```python
from build123d import *

# Parameters (mm, degrees)
BOSS_EXTRUDE1_DEPTH  = 1.5875
M8_CLEARANCE_HOLE1_D = 8.4


with BuildPart() as part:
    # Sketch1 → Boss-Extrude1 (new body)
    with BuildSketch(Plane(origin=(0, 0, 0), x_dir=(0, 0, -1), z_dir=(1, 0, 0))):
        with BuildLine():
            Line((-9.466844547, 1.05094211), (-8.132830894, 13.067683806))
            Line((-8.132830894, 13.067683806), (-6.55502347, 12.892526787))
            Line((-6.55502347, 12.892526787), (-4.453139249, 31.826215882))
            Line((-4.453139249, 31.826215882), (-6.030946674, 32.0013729))
            Line((-6.030946674, 32.0013729), (-4.696933021, 44.018114595))
            Line((-4.696933021, 44.018114595), (30.078862848, 47.728850174))
            ThreePointArc((30.078862848, 47.728850174), (38.60002065, 37.058807525), (51.869269545, 40.281690423))
            Line((51.869269545, 40.281690423), (35.966414021, 23.714419941))
            Line((35.966414021, 23.714419941), (34.821152107, 24.813752193))
            Line((34.821152107, 24.813752193), (21.629165093, 11.070609225))
            Line((21.629165093, 11.070609225), (22.774427007, 9.971276974))
            Line((22.774427007, 9.971276974), (6.871571484, -6.595993507))
            ThreePointArc((6.871571484, -6.595993507), (-4.037668467, -8.626868397), (-9.466844547, 1.05094211))
        make_face()
    extrude(amount=BOSS_EXTRUDE1_DEPTH)

    # M8 Clearance Hole1 (through all)
    with Locations(Plane(origin=(1.5875, 0, 0), x_dir=(0, 0, -1), z_dir=(1, 0, 0))):
        with Locations((0, 0)):
            Hole(M8_CLEARANCE_HOLE1_D / 2)


solid = part.part
```
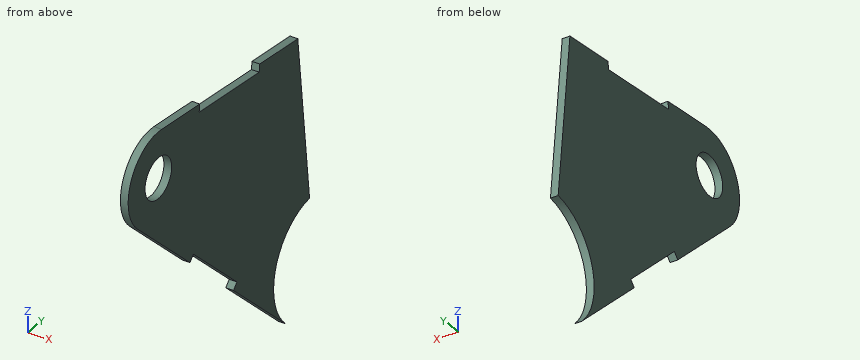
Build history of the part. All positions in model axes, mm. Give positions to 0.01 mm unless a question says otherwise; leave off trailing zeros. Loops run counter-clockwise (first coordinate to the right, second up) from the corner with the lowest first, then second, coordinate; pieces in that order, holes last. Notation, with made-up numbers: (12.25, 63.25) - (55.25, 63.25) arc R33 ccw to (55.25, 101.25) - close; hole circle Ø10 at (12.5, 3). An arc over 180 degrees is marked (long way). Use a Markdown table: item, result.
(1) Wall check: line 1 along Z through (x, y) = (1.5, -2); line 2 along Y through (x, z) = (1.05, 0) (3 decimals); line 3 along Z through (x, y) = (0.7, 34.5). Give the ranges that are in metal, low to high.
Taken from the geometry:
| item | result |
|---|---|
| line 1 | -11.28 to -3.69, 3.69 to 9.31 |
| line 2 | -9.525 to -4.2, 4.2 to 44.519 |
| line 3 | -46.32 to 5.75 |
(2) Band-saw the part on C-C (y = 0). Give the cut face in (x, z) (1 decimal).
Taken from the geometry:
| item | result |
|---|---|
| outline | (0, -13.2) - (1.6, -13.2) - (1.6, -4.2) - (0, -4.2) - close; (0, 4.2) - (1.6, 4.2) - (1.6, 9.5) - (0, 9.5) - close |
(3) Drop a flat-ended pin along its axis: pin 1 Ø1.5 at (y, z) = (13.5, -20) entering from -X. Give the stop position or say it passes through.
Taken from the geometry:
| item | result |
|---|---|
| pin 1 | x = 0 |
(4) Band-saw the part on B-B (z = 0). Give the cut face in (x, y) (1 decimal), and give its area (3 significant figures).
Taken from the geometry:
| item | result |
|---|---|
| outline | (0, -9.5) - (1.6, -9.5) - (1.6, -4.2) - (0, -4.2) - close; (0, 4.2) - (1.6, 4.2) - (1.6, 44.5) - (0, 44.5) - close |
| area | 72.5 mm2 |
(5) Band-saw the part on D-D (y = 19.5). Give the cut face in (x, z).
Taken from the geometry:
| item | result |
|---|---|
| outline | (0, -29.72) - (1.59, -29.72) - (1.59, 5.82) - (0, 5.82) - close |
(6) Band-saw the part on A-A (x = 1.3). Give the cut face in (y, z) (3 decimals).
Taken from the geometry:
| item | result |
|---|---|
| outline | (-6.596, -6.872) - (9.971, -22.774) - (11.071, -21.629) - (24.814, -34.821) - (23.714, -35.966) - (40.282, -51.869) arc R12.7 cw to (47.729, -30.079) - (44.018, 4.697) - (32.001, 6.031) - (31.826, 4.453) - (12.893, 6.555) - (13.068, 8.133) - (1.051, 9.467) arc R9.525 ccw to start; hole circle Ø8.4 at (0, 0) |
